The listing builds one solid part. Answer for the finished solid, in the listing's coordinates (mm). A direction names the side the tool comes from. Coordinates: 2 decimals unless noted, no trailing zeros. Write each loop counter-clockwise with the first axis right and the second up, starting at its lowest first coordinate (ties: lowest second). Pieces come first, ordered by that corner, then holes.
from build123d import *

# Parameters (mm, degrees)
ESBO_O1_W                = 1.6
ESBO_O1_H                = 99.6
RESSALTO_EXTRUS_O1_DEPTH = 230
ESBO_O2_W                = 1.6
ESBO_O2_H                = 99.6
RESSALTO_EXTRUS_O2_DEPTH = 232.5
ESBO_O5_W                = 97.5
ESBO_O5_H                = 42.5020002
CORTE_EXTRUS_O1_DEPTH    = 230
ESBO_O3_W                = 216
ESBO_O3_H                = 106.0040004
CORTE_EXTRUS_O2_DEPTH    = 2
ESBO_O8_R                = 2
CORTE_EXTRUS_O3_DEPTH    = 1


with BuildPart() as part:
    # Esboço1 → Ressalto-extrusão1 (new body)
    with BuildSketch(Plane.XY):
        with BuildLine():
            Line((-2.7, -61.339745962), (-2.7, 61.339745962))
            ThreePointArc((-2.7, 61.339745962), (-0.288049674, 60.341775891), (2.3, 60.0020002))
            Line((2.3, 60.0020002), (2.3, -60.0020002))
            ThreePointArc((2.3, -60.0020002), (-0.288049674, -60.341775891), (-2.7, -61.339745962))
        make_face()
        with Locations((-0.2, 0.2)):
            Rectangle(ESBO_O1_W, ESBO_O1_H, mode=Mode.SUBTRACT)
    extrude(amount=RESSALTO_EXTRUS_O1_DEPTH)

    # Esboço2 → Ressalto-extrusão2 (add)
    with BuildSketch(Plane.XY.offset(230)):
        with Locations((-0.2, 0.2)):
            Rectangle(ESBO_O2_W, ESBO_O2_H)
    extrude(amount=-RESSALTO_EXTRUS_O2_DEPTH)

    # Esboço5 → Corte-extrusão1 (cut)
    with BuildSketch(Plane(origin=(2.3, 0, 0), x_dir=(0, 0, -1), z_dir=(1, 0, 0))):
        with Locations((-167.25, 24.7510001)):
            Rectangle(ESBO_O5_W, ESBO_O5_H)
        with Locations((-62.75, 24.7510001)):
            Rectangle(ESBO_O5_W, ESBO_O5_H)
        with Locations((-167.25, -24.7510001)):
            Rectangle(ESBO_O5_W, ESBO_O5_H)
        with Locations((-62.75, -24.7510001)):
            Rectangle(ESBO_O5_W, ESBO_O5_H)
    extrude(amount=-CORTE_EXTRUS_O1_DEPTH, mode=Mode.SUBTRACT)

    # Esboço3 → Corte-extrusão2 (cut)
    with BuildSketch(Plane(origin=(2.3, 0, 0), x_dir=(0, 0, -1), z_dir=(1, 0, 0))):
        with Locations((-115, 0)):
            Rectangle(ESBO_O3_W, ESBO_O3_H)
    extrude(amount=-CORTE_EXTRUS_O2_DEPTH, mode=Mode.SUBTRACT)

    # Esboço8 → Corte-extrusão3 (cut)
    with BuildSketch(Plane(origin=(0.3, 0, 0), x_dir=(0, 0, -1), z_dir=(1, 0, 0))):
        with Locations(Location((-219, 49, 0), (0, 0, 90))):
            Circle(ESBO_O8_R)
        with Locations(Location((-11, 49, 0), (0, 0, 90))):
            Circle(ESBO_O8_R)
        with Locations(Location((-11, -49, 0), (0, 0, 90))):
            Circle(ESBO_O8_R)
        with Locations(Location((-219, -49, 0), (0, 0, 90))):
            Circle(ESBO_O8_R)
    extrude(amount=-CORTE_EXTRUS_O3_DEPTH, mode=Mode.SUBTRACT)


solid = part.part
Q1. Given pin 1 (2.5 mm diameter, centred on x = -1.5, y = -16.5, fed in from -Z); pin 2 (1.5 mm diameter, centred on x = 0.5, z = 40.5, fed in from +Y); pin 3 (4.5 mm diameter, centred on y = 49, z = 11, fed in from +X); pin 4 (0.9 mm diameter, centred on x = -1.5, z = 63.5, fed in from -Y), each flat-ended and moving along its own axis, determine where each tip first touches the part or whether it passes through.
Answers below:
pin 1: stops at z = -2.5
pin 2: stops at y = 60.33
pin 3: stops at x = 0.3
pin 4: stops at y = -60.95
Q2. The part is cut by section A-A, the plane y = -22.5. Write down the section's boundary in (x, z).
Answers below:
outline: (-2.7, 0) - (-1, 0) - (-1, -2.5) - (0.6, -2.5) - (0.6, 0) - (2.3, 0) - (2.3, 7) - (0.3, 7) - (0.3, 14) - (-2.7, 14) - close; (-2.7, 111.5) - (0.3, 111.5) - (0.3, 118.5) - (-2.7, 118.5) - close; (-2.7, 216) - (0.3, 216) - (0.3, 223) - (2.3, 223) - (2.3, 230) - (-2.7, 230) - close
Q3. The part is cut by section C-C, the plane x = -1.85. Write down the section's boundary in (y, z).
Answers below:
outline: (-60.9, 0) - (60.9, 0) - (60.9, 230) - (-60.9, 230) - close; hole (-46, 14) - (-3.5, 14) - (-3.5, 111.5) - (-46, 111.5) - close; hole (-46, 118.5) - (-3.5, 118.5) - (-3.5, 216) - (-46, 216) - close; hole (3.5, 14) - (46, 14) - (46, 111.5) - (3.5, 111.5) - close; hole (3.5, 118.5) - (46, 118.5) - (46, 216) - (3.5, 216) - close
Q4. Determine the mould class of faces 3 (the face through (0, 1, 230)), 4 (the face through (-0.7, 49, 219)), 5 (the face through (-0.25, -60.33, 113.39)) for opening direction Z: released by +Z, released by -Z, zero draft, split by the parting line, or undercut.
Answers below:
face 3: released by +Z
face 4: undercut
face 5: zero draft
Q5. The part is cut by section B-B, the plane z = 65. Write down the section's boundary in (x, y), then the cut area to 3 significant figures.
Answers below:
outline: (-2.7, -61.34) arc R10 cw to (2.3, -60) - (2.3, -53) - (0.3, -53) - (0.3, -46) - (-2.7, -46) - close; (-2.7, -3.5) - (0.3, -3.5) - (0.3, 3.5) - (-2.7, 3.5) - close; (-2.7, 46) - (0.3, 46) - (0.3, 53) - (2.3, 53) - (2.3, 60) arc R10 cw to (-2.7, 61.34) - close
area: 137 mm2
Q6. Find the intervals of material crossed by probe 1 along Z at (x, y) = (0.05, 6.5); probe 2 along Z at (x, y) = (-1.5, -13); probe 3 along Y at (x, z) = (-0.4, 219), in increasing order.
Answers below:
probe 1: z = -2.5 to 14, 111.5 to 118.5, 216 to 230
probe 2: z = 0 to 14, 111.5 to 118.5, 216 to 230
probe 3: y = -60.37 to -51, -47 to 47, 51 to 60.37
Q7. The part is cut by section D-D, the plane z = 115.5. Write down the section's boundary in (x, y), then the cut area to 3 significant figures.
Answers below:
outline: (-2.7, -61.34) arc R10 cw to (2.3, -60) - (2.3, -53) - (0.3, -53) - (0.3, 53) - (2.3, 53) - (2.3, 60) arc R10 cw to (-2.7, 61.34) - close
area: 392 mm2
Q8. Which of the six approach directions +Z, -Z, +X, -X, +Y, -Y give full straight-line access (tool end or side, diameter ignored) to faces 1 (the face through (-0.7, 49, 11)), 2 (the face through (2.3, 54, 106))?
Answers below:
face 1: +X
face 2: +Z, -Z, +X, +Y, -Y
